The model under review builds one solid part; all positions refer to its coordinate system, in mm. Coordinates: 2 decimals unless noted, no trailing zeros. Write each loop counter-clockwise with the first axis right and the second up, starting at its lowest first coordinate (ties: lowest second). Pieces come first, ordered by that corner, then holes. Notation, with made-up numbers: (34.25, 22.25) -> (40.25, 22.25) arc R19 ccw to (40.25, 37.25) -> close; hole circle Ø1 at (-23, 78.25). An arc over 180 degrees is marked (long way). Put each result on its own line as item: value. Start each with the question number.
from build123d import *

# Parameters (mm, degrees)
SKETCH1_R               = 65
SKETCH1_R_2             = 62.5
BOSS_EXTRUDE1_DEPTH     = 587.5
CUT_EXTRUDE1_DEPTH      = 37.5
CUT_EXTRUDE1_DEPTH_BACK = 312.5
FILLET1_R               = 10
SKETCH5_R               = 2
CUT_EXTRUDE2_DEPTH      = 100
SKETCH6_R               = 2
CUT_EXTRUDE3_DEPTH      = 135.5


with BuildPart() as part:
    # Sketch1 → Boss-Extrude1 (new, symmetric)
    with BuildSketch(Plane(origin=(0, 0, 0), x_dir=(0, 0, -1), z_dir=(1, 0, 0))):
        Circle(SKETCH1_R)
        Circle(SKETCH1_R_2, mode=Mode.SUBTRACT)
    extrude(amount=BOSS_EXTRUDE1_DEPTH, both=True)

    # Sketch3 → Cut-Extrude1 (cut, two sides: drawn at the far end of the back side and taken through both)
    with BuildSketch(Plane(origin=(0, 0, 0), x_dir=(0, 0, -1), z_dir=(1, 0, 0)).offset(-CUT_EXTRUDE1_DEPTH_BACK)):
        with BuildLine():
            Line((-56.291651246, 32.5), (-54.126587737, 31.25))
            ThreePointArc((-54.126587737, 31.25), (0, 62.5), (54.126587737, 31.25))
            Line((54.126587737, 31.25), (56.291651246, 32.5))
            ThreePointArc((56.291651246, 32.5), (0, 65), (-56.291651246, 32.5))
        make_face()
    extrude(amount=CUT_EXTRUDE1_DEPTH + CUT_EXTRUDE1_DEPTH_BACK, mode=Mode.SUBTRACT)

    # Fillet1
    fillet1_edges = [part.edges().sort_by_distance(p)[0] for p in [
        (-312.5, 31.875, 55.209119491),
        (-312.5, 31.875, -55.209119491),
        (37.5, 31.875, 55.209119491),
        (37.5, 31.875, -55.209119491),
    ]]
    fillet(fillet1_edges, radius=FILLET1_R)

    # Sketch5 → Cut-Extrude2 (cut, symmetric)
    with BuildSketch(Plane(origin=(0, 0, 0), x_dir=(1, 0, 0), z_dir=(0, 1, 0))):
        with Locations(Location((-318.5, 0, 0), (0, 0, 270))):
            Circle(SKETCH5_R)
        with Locations(Location((42.5, 0, 0), (0, 0, 270))):
            Circle(SKETCH5_R)
    extrude(amount=CUT_EXTRUDE2_DEPTH, both=True, mode=Mode.SUBTRACT)

    # Sketch6 → Cut-Extrude3 (cut, symmetric)
    with BuildSketch(Plane.XY):
        with Locations((-318.5, 0)):
            Circle(SKETCH6_R)
        with Locations((42.5, 0)):
            Circle(SKETCH6_R)
    extrude(amount=CUT_EXTRUDE3_DEPTH, both=True, mode=Mode.SUBTRACT)


solid = part.part
1. Consider section C-C on x = 95.5. State the section outline as (y, z) points, then the cut area to 3 significant figures.
2. Consider section B-B on z = 34.5. State the section outline as (x, y) points, then the cut area to 3 significant figures.
3. The part is to be moulded in two halves that separate along X. For faces 1 (the flat face through (587.5, 53, 34)), 2 (the flat face through (37.5, 63, 0)), 3 (the flat face through (-312.5, 63, 0)), 4 (the cylindrical face through (8.225, -63.454, 14.091)), say which applies: released by +X, released by -X, zero draft, split by the parting line, or undercut.
4. Consider section D-D on y = 21.5. State the section outline as (x, z) points, then the cut area to 3 significant figures.
5. Insertion check: P1, Ø12, axis at x = -231.5, z = 6.5, coming from the -Y side; P2, Ø10, axis at x = -334, z = -45, coming from the -Y side; P3, Ø4, axis at x = -369, z = 39, coming from the +Y side; P4, Ø1, axis at x = 266, z = -4.5, coming from the -Y side. Each pin has a flat end and moves straight along its axis. Give the tip position at first contact, or say it passes through.
6. Wall thickness on line 1 (X direction, y = -64.2, z = 0); line 2 (Y direction, x = 64, z = 0); line 3 (Z direction, x = 381, y = 1): over which ranges is each line inside the solid? List them lowest first. Write a range as from..to.
7. Consider section A-A on y = -24.5. State the section outline as (x, z) points, then the cut area to 3 significant figures.
Output values:
1. outline: circle Ø130 at (0, 0); hole circle Ø125 at (0, 0)
1. area: 1,000 mm^2
2. outline: (-587.5, -55.09) -> (587.5, -55.09) -> (587.5, -52.12) -> (-587.5, -52.12) -> close; (-587.5, 52.12) -> (-312.5, 52.12) -> (-312.5, 55.09) -> (-587.5, 55.09) -> close; (37.5, 52.12) -> (587.5, 52.12) -> (587.5, 55.09) -> (37.5, 55.09) -> close
2. area: 5,950 mm^2
3. face 1: released by +X
3. face 2: undercut
3. face 3: undercut
3. face 4: zero draft
4. outline: (-587.5, -61.34) -> (587.5, -61.34) -> (587.5, -58.69) -> (-587.5, -58.69) -> close; (-587.5, 58.69) -> (587.5, 58.69) -> (587.5, 61.34) -> (-587.5, 61.34) -> close
4. area: 6,240 mm^2
5. P1: stops at y = -65
5. P2: stops at y = -51.23
5. P3: stops at y = 53.44
5. P4: stops at y = -64.88
6. line 1: x = -587.5..-320.5, -316.5..40.5, 44.5..587.5
6. line 2: y = -65..-62.5, 62.5..65
6. line 3: z = -64.99..-62.49, 62.49..64.99
7. outline: (-587.5, -60.21) -> (587.5, -60.21) -> (587.5, -57.5) -> (-587.5, -57.5) -> close; (-587.5, 57.5) -> (587.5, 57.5) -> (587.5, 60.21) -> (-587.5, 60.21) -> close
7. area: 6,360 mm^2
